Autodesk Inventor part; units mm, degrees
ref_plane "YZ Plane" through (0, 0, 0) normal (1, 0, 0) x (0, 1, 0)
ref_plane "XZ Plane" through (0, 0, 0) normal (0, 1, 0) x (-1, 0, 0)
ref_plane "XY Plane" through (0, 0, 0) normal (0, 0, 1) x (1, 0, 0)
sketch "Sketch1" plane through (0, 0, 0) normal (0, 0, 1) x (1, 0, 0)
  circle A0 centre (0, 0) radius 600
  circle A1 centre (0, 0) radius 575
  circle A2 centre (0, 0) radius 525
  dimension "d0" = 1200
  dimension "d3" = 1150
  dimension "d4" = 1050
extrude "Extrusion1" add sketch "Sketch1" along normal blind 50 contours A0 | A1 | A2
extrude "Extrusion2" cut sketch "Sketch1" along normal blind 20 contours A1
sketch "Sketch2" plane through (0, 0, 50) normal (0, 0, 1) x (1, 0, 0)
  line L0 (0, 0) -> (0, 350) construction
  line L1 (0, 350) -> (-255.3075, 350) construction
  line L2 (-259.8075, 350) -> (255.3075, 350)
  line L3 (259.8075, 345.5) -> (259.8075, 154.5)
  line L4 (255.3075, 150) -> (-257.8075, 150)
  line L5 (-259.8075, 152) -> (-259.8075, 345.5)
  arc A0 (-259.8075, 152) -> (-257.8075, 150) centre (-257.8075, 152) ccw
  arc A1 (-255.3075, 350) -> (-259.8075, 345.5) centre (-255.3075, 345.5) ccw
  arc A2 (259.8075, 345.5) -> (255.3075, 350) centre (255.3075, 345.5) ccw
  arc A3 (255.3075, 150) -> (259.8075, 154.5) centre (255.3075, 154.5) ccw
  line L6 (-259.8075, 150) -> (-259.8075, 154.5) construction
  line L7 (-259.8075, 154.5) -> (-255.3075, 154.5) construction
  line L8 (255.3075, 350) -> (255.3075, 345.5) construction
  line L9 (250.8075, 345.5) -> (-250.8075, 345.5)
  line L10 (-255.3075, 341) -> (-255.3075, 159)
  line L11 (-250.8075, 154.5) -> (250.8075, 154.5)
  line L12 (255.3075, 159) -> (255.3075, 341)
  arc A4 (-255.3075, 159) -> (-250.8075, 154.5) centre (-250.8075, 159) ccw
  arc A5 (-250.8075, 345.5) -> (-255.3075, 341) centre (-250.8075, 341) ccw
  arc A6 (255.3075, 341) -> (250.8075, 345.5) centre (250.8075, 341) ccw
  arc A7 (250.8075, 154.5) -> (255.3075, 159) centre (250.8075, 159) ccw
  point P0 (259.8075, 350)
  dimension "d7" = 350
  dimension "d8" = 259.8075
  dimension "d9" = 519.615
  dimension "d10" = 200
  dimension "d11" = 2
  dimension "d12" = 4.5
  dimension "d13" = 4.5
  dimension "d14" = 4.5
  dimension "d15" = 4.5
extrude "Extrusion3" cut sketch "Sketch2" against normal through all contours A6 L12 A7 L11 A4 L10 A5 L9
extrude "Extrusion4" cut sketch "Sketch2" against normal blind 25
properties part number "Base Plate"
Input: part model. Units: mm. Frame: model coordinates. A direction names the side the tool comes from. Give positions to 0.01 mm unless a question says otherwise; leave off trailing zeros. Loops run counter-clockwise (first coordinate to the right, second up) from the corner with the lowest first, then second, coordinate; pieces in that order, holes last. Notation, with made-up numbers: (3, 58.25) -> (49, 58.25) arc R18 ccw to (49, 93.25) -> close; hole circle Ø10 at (85, 84.5). An arc over 180 degrees is marked (long way). Use a Markdown table: item, result.
Q1. Section query C-C, the plane z = 37.5. Return the cut outline in (x, y).
Entries:
| item | result |
|---|---|
| outline | circle Ø1200 at (0, 0); hole (-259.81, 152) arc R2 ccw to (-257.81, 150) -> (255.31, 150) arc R4.5 ccw to (259.81, 154.5) -> (259.81, 345.5) arc R4.5 ccw to (255.31, 350) -> (-255.31, 350) arc R4.5 ccw to (-259.81, 345.5) -> close |
Q2. First-contact query: P1, Ø12.5, axis at x = 68, z = 17.5, coming from the -Y side; P2, Ø20, axis at x = -121.5, z = 40.5, coming from the -Y side; P3, Ø12, axis at x = -252, z = 23.5, coming from the +Y side. Flat tips, straight axial feed; report the tip coordinate or a pass-through.
Entries:
| item | result |
|---|---|
| P1 | stops at y = -596.81 |
| P2 | stops at y = -589.55 |
| P3 | stops at y = 547.25 |
Q3. Access query for faces 1 (the cylindrical face through (-574.444, -25.282, 9.86)), 2 (the flat face through (-8, 8, 50)). Directions: +Z, -Z, +X, -X, +Y, -Y. A direction counts if a zero-diameter tool reaches every point of the face in a straight line with its end or side. Return the directions, or none.
Entries:
| item | result |
|---|---|
| face 1 | -Z |
| face 2 | +Z, +X, -X, +Y, -Y |
Q4. Section query A-A, the plane x = 0. Return the cut outline in (y, z), plus the area to 3 significant figures.
Entries:
| item | result |
|---|---|
| outline | (-600, 0) -> (-575, 0) -> (-575, 20) -> (-525, 20) -> (-525, 0) -> (154.5, 0) -> (154.5, 25) -> (150, 25) -> (150, 50) -> (-600, 50) -> close; (345.5, 0) -> (525, 0) -> (525, 20) -> (575, 20) -> (575, 0) -> (600, 0) -> (600, 50) -> (350, 50) -> (350, 25) -> (345.5, 25) -> close |
| area | 48,200 mm² |
Q5. Ray query, probe 1 along Y at (x, z) = (6, 17); probe 2 along X at (y, z) = (212.5, 10.5); probe 3 along X at (y, z) = (-414.5, 16.5). Return the intervals inside material, ascending. Write a range as from..to.
Entries:
| item | result |
|---|---|
| probe 1 | y = -599.97..-574.97, -524.97..154.5, 345.5..524.97, 574.97..599.97 |
| probe 2 | x = -561.11..-534.29, -480.07..-255.31, 255.31..480.07, 534.29..561.11 |
| probe 3 | x = -433.81..-398.52, -322.2..322.2, 398.52..433.81 |
Q6. Section query D-D, the plane y = 0. Return the cut outline in (x, z).
Entries:
| item | result |
|---|---|
| outline | (-600, 0) -> (-575, 0) -> (-575, 20) -> (-525, 20) -> (-525, 0) -> (525, 0) -> (525, 20) -> (575, 20) -> (575, 0) -> (600, 0) -> (600, 50) -> (-600, 50) -> close |
Q7. Section query B-B, the plane y = 198. Return the cut outline in (x, z).
Entries:
| item | result |
|---|---|
| outline | (-566.39, 0) -> (-539.83, 0) -> (-539.83, 20) -> (-486.23, 20) -> (-486.23, 0) -> (-255.31, 0) -> (-255.31, 25) -> (-259.81, 25) -> (-259.81, 50) -> (-566.39, 50) -> close; (255.31, 0) -> (486.23, 0) -> (486.23, 20) -> (539.83, 20) -> (539.83, 0) -> (566.39, 0) -> (566.39, 50) -> (259.81, 50) -> (259.81, 25) -> (255.31, 25) -> close |
Q8. Pull-direction query (X, two-part tool) for faces 3 (the flat face through (-1, 154, 25)), 4 (the cylindrical face through (-78.108, -594.894, 24.65)), 5 (the flat face through (486, -308, 0)); classes: pulls with the +X half, pulls with the -X half, needs draft (parallel to the pull), parting line crosses it, or undercut.
Entries:
| item | result |
|---|---|
| face 3 | undercut |
| face 4 | parting line crosses it |
| face 5 | needs draft |
